from build123d import *

# Parameters (mm, degrees)
SKETCH1_W                      = 35
SKETCH1_H                      = 60
BOSS_EXTRUDE1_DEPTH            = 5.4
CUT_EXTRUDE1_REACH             = 37.148
SKETCH2_W                      = 35
SKETCH2_H                      = 2.655
SKETCH2_R                      = 2
SKETCH2_H_2                    = 17.637243623
SKETCH2_H_3                    = 9.707756377
CUT_EXTRUDE1_DIRECTION_2_DEPTH = 36.148399679


with BuildPart() as part:
    # Sketch1 → Boss-Extrude1 (new body)
    with BuildSketch(Plane.XY):
        Rectangle(SKETCH1_W, SKETCH1_H)
    extrude(amount=BOSS_EXTRUDE1_DEPTH)

    # Sketch2 → Cut-Extrude1 (cut, up to next)
    with BuildSketch(Plane.XY.offset(5.4), mode=Mode.PRIVATE) as cut_extrude1_sk1:
        with Locations((0, 28.6725)):
            Rectangle(SKETCH2_W, SKETCH2_H)
    cut_extrude1_tool1 = extrude(cut_extrude1_sk1.sketch, amount=-CUT_EXTRUDE1_REACH, mode=Mode.PRIVATE) & part.part
    # Sketch2 → Cut-Extrude1 (cut, up to next)
    with BuildSketch(Plane.XY.offset(5.4), mode=Mode.PRIVATE) as cut_extrude1_sk2:
        with Locations(Location((-10, 19.84, 0), (0, 0, 180))):
            Circle(SKETCH2_R)
    cut_extrude1_tool2 = extrude(cut_extrude1_sk2.sketch, amount=-CUT_EXTRUDE1_REACH, mode=Mode.PRIVATE) & part.part
    # Sketch2 → Cut-Extrude1 (cut, up to next)
    with BuildSketch(Plane.XY.offset(5.4), mode=Mode.PRIVATE) as cut_extrude1_sk3:
        with Locations(Location((10, 19.84, 0), (0, 0, 180))):
            Circle(SKETCH2_R)
    cut_extrude1_tool3 = extrude(cut_extrude1_sk3.sketch, amount=-CUT_EXTRUDE1_REACH, mode=Mode.PRIVATE) & part.part
    # Sketch2 → Cut-Extrude1 (cut, up to next)
    with BuildSketch(Plane.XY.offset(5.4), mode=Mode.PRIVATE) as cut_extrude1_sk4:
        with Locations(Location((-10, 4.84, 0), (0, 0, 180))):
            Circle(SKETCH2_R)
    cut_extrude1_tool4 = extrude(cut_extrude1_sk4.sketch, amount=-CUT_EXTRUDE1_REACH, mode=Mode.PRIVATE) & part.part
    # Sketch2 → Cut-Extrude1 (cut, up to next)
    with BuildSketch(Plane.XY.offset(5.4), mode=Mode.PRIVATE) as cut_extrude1_sk5:
        with Locations(Location((10, 4.84, 0), (0, 0, 180))):
            Circle(SKETCH2_R)
    cut_extrude1_tool5 = extrude(cut_extrude1_sk5.sketch, amount=-CUT_EXTRUDE1_REACH, mode=Mode.PRIVATE) & part.part
    # Sketch2 → Cut-Extrude1 (cut, up to next)
    with BuildSketch(Plane.XY.offset(5.4), mode=Mode.PRIVATE) as cut_extrude1_sk6:
        with Locations((0, -11.473621812)):
            Rectangle(SKETCH2_W, SKETCH2_H_2)
    cut_extrude1_tool6 = extrude(cut_extrude1_sk6.sketch, amount=-CUT_EXTRUDE1_REACH, mode=Mode.PRIVATE) & part.part
    # Sketch2 → Cut-Extrude1 (cut, up to next)
    with BuildSketch(Plane.XY.offset(5.4), mode=Mode.PRIVATE) as cut_extrude1_sk7:
        with Locations((0, -25.146121812)):
            Rectangle(SKETCH2_W, SKETCH2_H_3)
    cut_extrude1_tool7 = extrude(cut_extrude1_sk7.sketch, amount=-CUT_EXTRUDE1_REACH, mode=Mode.PRIVATE) & part.part
    add(cut_extrude1_tool1.solids().sort_by_distance((0, 28.6725, 5.4))[0], mode=Mode.SUBTRACT)
    add(cut_extrude1_tool2.solids().sort_by_distance((-10, 19.84, 5.4))[0], mode=Mode.SUBTRACT)
    add(cut_extrude1_tool3.solids().sort_by_distance((10, 19.84, 5.4))[0], mode=Mode.SUBTRACT)
    add(cut_extrude1_tool4.solids().sort_by_distance((-10, 4.84, 5.4))[0], mode=Mode.SUBTRACT)
    add(cut_extrude1_tool5.solids().sort_by_distance((10, 4.84, 5.4))[0], mode=Mode.SUBTRACT)
    add(cut_extrude1_tool6.solids().sort_by_distance((0, -11.473622, 5.4))[0], mode=Mode.SUBTRACT)
    add(cut_extrude1_tool7.solids().sort_by_distance((0, -25.146122, 5.4))[0], mode=Mode.SUBTRACT)

    # Sketch2 → Cut-Extrude1 direction 2 (cut)
    with BuildSketch(Plane.XY.offset(5.4)):
        with Locations((0, 28.6725)):
            Rectangle(SKETCH2_W, SKETCH2_H)
        with Locations(Location((-10, 19.84, 0), (0, 0, 180))):
            Circle(SKETCH2_R)
        with Locations(Location((10, 19.84, 0), (0, 0, 180))):
            Circle(SKETCH2_R)
        with Locations(Location((-10, 4.84, 0), (0, 0, 180))):
            Circle(SKETCH2_R)
        with Locations(Location((10, 4.84, 0), (0, 0, 180))):
            Circle(SKETCH2_R)
        with Locations((0, -11.473621812)):
            Rectangle(SKETCH2_W, SKETCH2_H_2)
        with Locations((0, -25.146121812)):
            Rectangle(SKETCH2_W, SKETCH2_H_3)
    extrude(amount=CUT_EXTRUDE1_DIRECTION_2_DEPTH, mode=Mode.SUBTRACT)


solid = part.part
Geometry check sheet. Reference: the model listing, model coordinates, mm. Give positions to 0.01 mm unless a question says otherwise; leave off trailing zeros. Loops run counter-clockwise (first coordinate to the right, second up) from the corner with the lowest first, then second, coordinate; pieces in that order, holes last. Notation, with made-up numbers: M 3,-29 L 17,-29 A26 cw 17,-9 Z; hole C 60.25,11.5 d7. An arc over 180 degrees is marked long. Answer as a JSON object with one key per item and string values. Group by question number.
Item 1: Gauge pin test, flat end, axial feed: pin 1 (6.5 mm diameter, centred on x = 10, y = 4.84, fed in from +Z). Record the tip position at first contact, or that the pin passes through.
Item 2: Sectioned sample at C-C on z = 4.95. Record the boundary of the cut face in (x, y) (3 decimals).
Item 3: Sectioned sample at B-B on x = 10. Record the boundary of the cut face in (y, z) (3 decimals).
Item 4: Mould release check, pull along X, two halves, no side actions. Record for faces 1 (the cylindrical face through (-9.74, 17.857, 2.738)), 2 (the flat face through (17.5, 12, 3)), 3 (the flat face through (0, -2.655, 3)), 4 (the cylindrical face through (10.26, 17.857, 2.738)): pulls with the +X half, pulls with the -X half, needs draft (parallel to the pull), parting line crosses it, or undercut.
Item 5: Material ranges on L1, parallel to X at y = 19.84, z = 2.3; L2, parallel to Y at x = 10, z = 2.9 (3 decimals); L3, parallel to Y at x = -8.5, z = 2.4 (3 decimals), recorded low to high.
Item 6: Sectioned sample at A-A on y = 4.84. Record the boundary of the cut face in (x, z), plus the area to 3 significant figures.
Findings below:
{
 "1": {"pin 1": "z = 5.4"},
 "2": {"outline": "M -17.5,-2.655 L 17.5,-2.655 L 17.5,27.345 L -17.5,27.345 Z; hole C -10,4.84 d4; hole C -10,19.84 d4; hole C 10,4.84 d4; hole C 10,19.84 d4"},
 "3": {"outline": "M -2.655,0 L 2.84,0 L 2.84,5.4 L -2.655,5.4 Z; M 6.84,0 L 17.84,0 L 17.84,5.4 L 6.84,5.4 Z; M 21.84,0 L 27.345,0 L 27.345,5.4 L 21.84,5.4 Z"},
 "4": {"face 1": "undercut", "face 2": "pulls with the +X half", "face 3": "needs draft", "face 4": "undercut"},
 "5": {"L1": "-17.5 to -12, -8 to 8, 12 to 17.5", "L2": "-2.655 to 2.84, 6.84 to 17.84, 21.84 to 27.345", "L3": "-2.655 to 3.517, 6.163 to 18.517, 21.163 to 27.345"},
 "6": {"outline": "M -17.5,0 L -12,0 L -12,5.4 L -17.5,5.4 Z; M -8,0 L 8,0 L 8,5.4 L -8,5.4 Z; M 12,0 L 17.5,0 L 17.5,5.4 L 12,5.4 Z", "area": "146 mm2"}
}
